For this review, use the dimensioned drawing (mm, ordinates from the lowest corner) and the shaded views. A direction names the side the tool comes from. Coordinates: 2 decimals unless noted, no trailing zeros. Write each loop counter-clockwise with the first axis right and the second up, starting at its lowest first coordinate (ties: lowest second). Pieces come first, ordered by that corner, then holes. Notation, with made-up numbers: (-35, 2) - (-6, 2) arc R24 cw to (-6, 13) - close; hole circle Ø8 at (55, 47). An arc over 180 degrees is marked (long way). One line per item, written item: value.
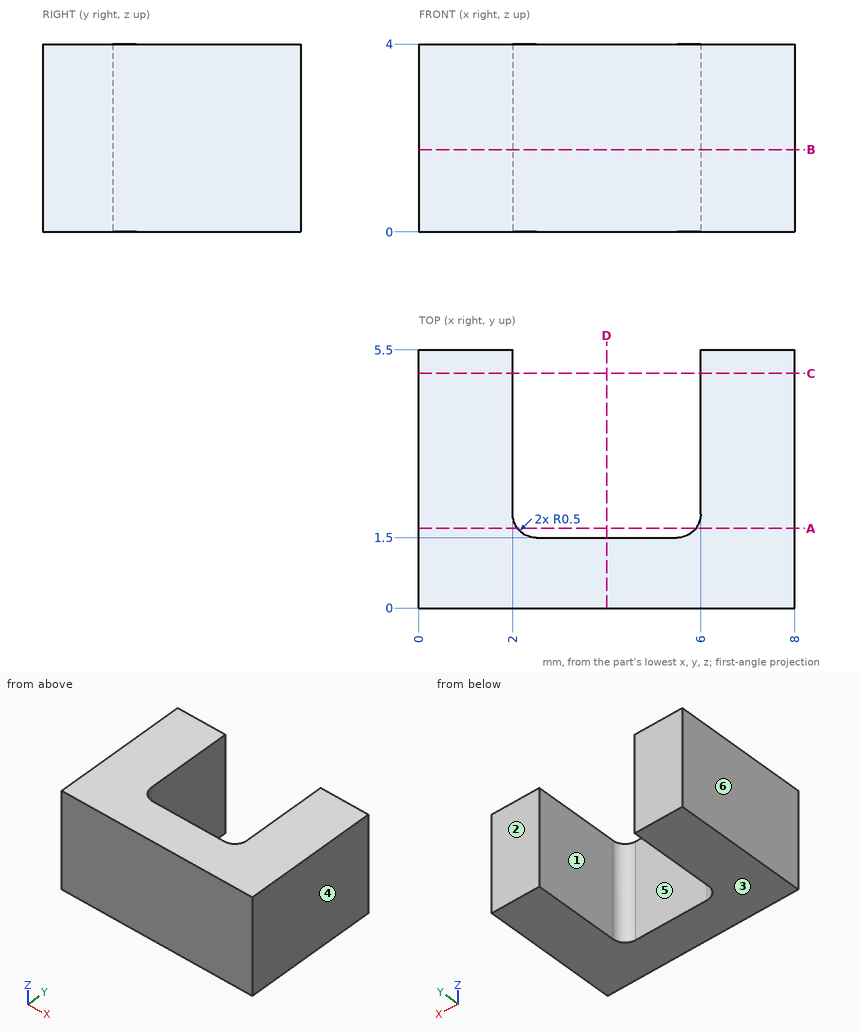
1. Consider section C-C, the plane y = 5. Write out the cut boundary in (x, z), then the cut area to 3 significant figures.
Answer block:
outline: (0, 0) - (2, 0) - (2, 4) - (0, 4) - close; (6, 0) - (8, 0) - (8, 4) - (6, 4) - close
area: 16.0 mm^2
2. Mouldability with a two-part tool opening along X and no side actions: class the marked faces 3, 4, 5 and 6 as released by +X, released by -X, zero draft, split by the parting line, or undercut.
Answer block:
face 3: zero draft
face 4: released by +X
face 5: undercut
face 6: released by -X
3. Wall thickness on line 1 along X through (y, z) = (5.2, 0.75); line 2 along Y through (x, z) = (2.75, 0.55): over which ranges is each line inside the solid? List them lowest first.
Answer block:
line 1: x = 0 to 2, 6 to 8
line 2: y = 0 to 1.5
4. Consider section B-B, the plane z = 1.75. Write out the cut boundary in (x, y), then the cut area to 3 significant figures.
Answer block:
outline: (0, 0) - (8, 0) - (8, 5.5) - (6, 5.5) - (6, 2) arc R0.5 cw to (5.5, 1.5) - (2.5, 1.5) arc R0.5 cw to (2, 2) - (2, 5.5) - (0, 5.5) - close
area: 28.1 mm^2
5. Consider section D-D, the plane x = 4. Write out the cut boundary in (y, z).
Answer block:
outline: (0, 0) - (1.5, 0) - (1.5, 4) - (0, 4) - close
6. Insertion check: pin 1 Ø2 at (x, z) = (5.5, 0.5) entering from +Y; pin 2 Ø0.9 at (x, z) = (4.5, 1) entering from +Y. Each pin has a flat end and moves straight along its axis. Give the tip position at first contact, or say it passes through.
Answer block:
pin 1: stops at y = 5.5
pin 2: stops at y = 1.5
7. For the marked faces 1 and 2, list the 3-axis set-ups (+Z, -Z, +X, -X, +Y, -Y) from which the entire face can be reached by the end or side of a thin tool; tool diameter is ignored.
Answer block:
face 1: +Z, -Z, +Y
face 2: +Z, -Z, +X, -X, +Y
8. Consider section A-A, the plane y = 1.7. Write out the cut boundary in (x, z), then the cut area to 3 significant figures.
Answer block:
outline: (0, 0) - (2.1, 0) - (2.1, 4) - (0, 4) - close; (5.9, 0) - (8, 0) - (8, 4) - (5.9, 4) - close
area: 16.8 mm^2
